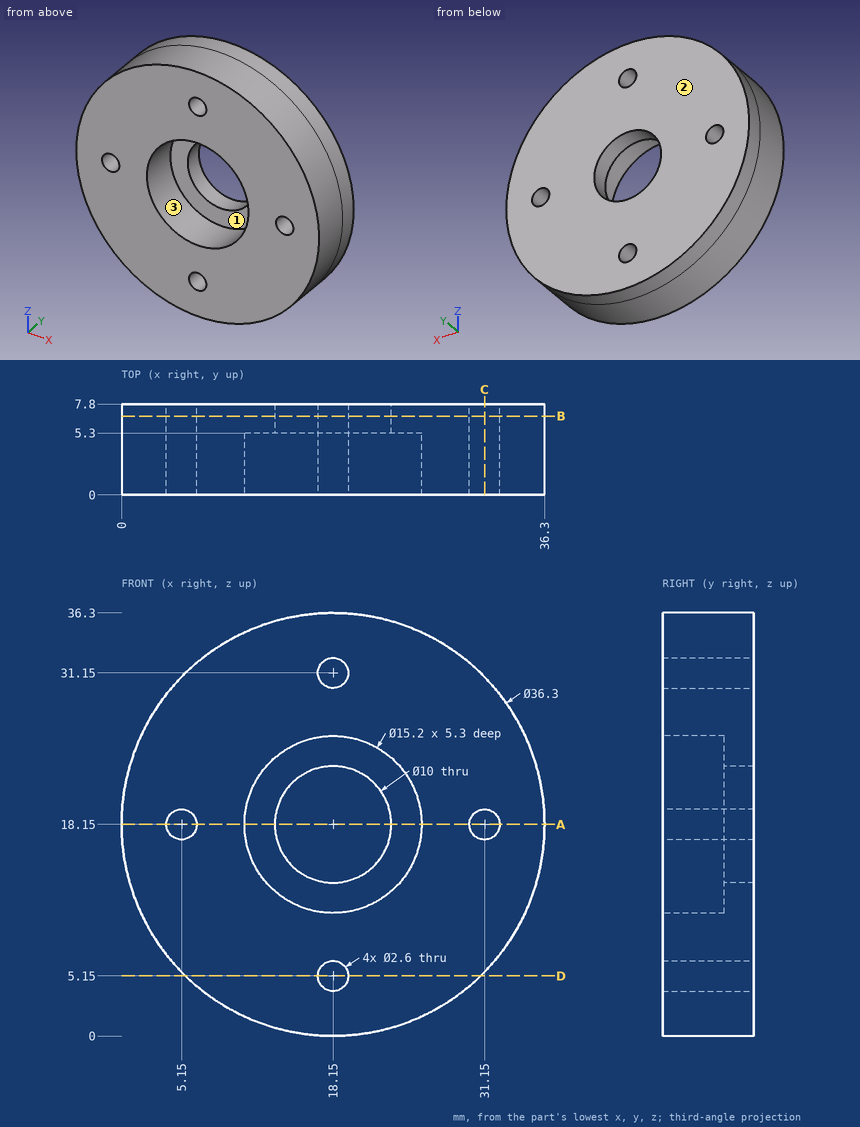
Job drawing, mm, ordinate dimensions from the low corner. One solid piece. Round coordinates to 2 decimals unless told otherwise and drop trailing zeros. Loops run counter-clockwise (first coordinate to the right, second up) from the corner with the lowest first, then second, coordinate; pieces in that order, holes last.
(1) Cut at B-B (y = 6.75). Give the cut face in (x, z).
(2) Cut at C-C (x = 31.15). Give the cut face in (y, z).
(3) Cut at D-D (z = 5.15). Give the cut face in (x, y), plus the area to 3 significant figures.
(4) Cut at A-A (z = 18.15). Give the cut face in (x, y).
(5) Two-plate mould, pull along X, no slides. Class the marked faces 1, 2 and 3: +X half, -X half, draft (parallel to the pull), parting line (faces both ways), or undercut.
(6) Drop flat-ended pins along their axis: pin 1 (1.5 mm diameter, centred on y = 2, z = 4.5, fed in from -X); pin 2 (3 mm diameter, centred on x = 18.5, y = 2.5, fed in from -Z); pin 3 (3 mm diameter, centred on y = 6, z = 16.5, fed in from -X). Give the stop position or say it passes through.
(7) Wall check: line 1 along X through (y, z) = (2.5, 18.15); line 2 along Z through (x, y) = (18.15, 5.5). Give the ranges that are in metal, low to high.
Findings below:
1. outline: circle Ø36.3 at (18.15, 18.15); hole circle Ø2.6 at (5.15, 18.15); hole circle Ø10 at (18.15, 18.15); hole circle Ø2.6 at (18.15, 5.15); hole circle Ø2.6 at (18.15, 31.15); hole circle Ø2.6 at (31.15, 18.15)
2. outline: (0, 5.48) - (7.8, 5.48) - (7.8, 16.85) - (0, 16.85) - close; (0, 19.45) - (7.8, 19.45) - (7.8, 30.82) - (0, 30.82) - close
3. outline: (5.48, 0) - (16.85, 0) - (16.85, 7.8) - (5.48, 7.8) - close; (19.45, 0) - (30.82, 0) - (30.82, 7.8) - (19.45, 7.8) - close
3. area: 177 mm2
4. outline: (0, 0) - (3.85, 0) - (3.85, 7.8) - (0, 7.8) - close; (6.45, 0) - (10.55, 0) - (10.55, 5.3) - (13.15, 5.3) - (13.15, 7.8) - (6.45, 7.8) - close; (23.15, 5.3) - (25.75, 5.3) - (25.75, 0) - (29.85, 0) - (29.85, 7.8) - (23.15, 7.8) - close; (32.45, 0) - (36.3, 0) - (36.3, 7.8) - (32.45, 7.8) - close
5. face 1: undercut
5. face 2: draft
5. face 3: undercut
6. pin 1: stops at x = 5.38
6. pin 2: stops at z = 0
6. pin 3: stops at x = 0
7. line 1: x = 0 to 3.85, 6.45 to 10.55, 25.75 to 29.85, 32.45 to 36.3
7. line 2: z = 0 to 3.85, 6.45 to 13.15, 23.15 to 29.85, 32.45 to 36.3
